from build123d import *

# Parameters (mm, degrees)
SKETCH1_R           = 38
BOSS_EXTRUDE1_DEPTH = 10
SKETCH2_R           = 2.5
CUT_EXTRUDE1_DEPTH  = 10
CIRPATTERN1_COUNT   = 8


with BuildPart() as part:
    # Sketch1 → Boss-Extrude1 (new body)
    with BuildSketch(Plane.XY):
        Circle(SKETCH1_R)
    extrude(amount=BOSS_EXTRUDE1_DEPTH)

    # Sketch2 → Cut-Extrude1 (cut)
    with BuildSketch(Plane(origin=(0, 38, 0), x_dir=(1, 0, 0), z_dir=(0, 1, 0))):
        with Locations((0, -5)):
            Circle(SKETCH2_R)
    cut_extrude1 = extrude(amount=-CUT_EXTRUDE1_DEPTH, mode=Mode.SUBTRACT)

    # CirPattern1: Cut-Extrude1 ×8 about axis
    cirpattern1_axis = Axis((0, 0, 0), (0, 0, 1))
    for i in range(1, CIRPATTERN1_COUNT):
        add(cut_extrude1.rotate(cirpattern1_axis, i * 360 / CIRPATTERN1_COUNT), mode=Mode.SUBTRACT)


solid = part.part
Verification items for the finished model (mm, model axes). A direction names the side the tool comes from. Give positions to 0.01 mm unless a question says otherwise; leave off trailing zeros. Order: outer loops, then holes, each group sorted by start corner. A loop starts at its lowest first (then second) coordinate and runs counter-clockwise, first axis right, second up. Notation, with made-up numbers: M 1,9.5 L 22,9.5 A17 ccw 22,35.5 Z; hole C 44,53 d8. An arc over 180 degrees is marked long. Answer as a JSON object with one key per item and string values. Group by question number.
1) Cross-section at A-A (y = 0). Enter the section's corners in (x, z), then the cut area to 3 significant figures.
2) Depth check by flat-ended pin: pin 1 Ø1.5 at (y, z) = (1, 4) entering from -X; pin 2 Ø2.5 at (x, z) = (0.5, 4.5) entering from +Y; pin 3 Ø5 at (x, z) = (15, 5.5) entering from -Y. Enter the tip coordinate at first touch or a pass-through.
3) Scan lines: line 1 along Z through (x, y) = (-31, 0); line 2 along X through (y, z) = (-33.5, 7.25); line 3 along Y through (x, z) = (-30.5, 2.75). Record each from-to range of solid material in increasing order. Write a range as [from, to].
4) Mould release check, pull along X, two halves, no side actions. Record for faces 1 (the face through (35.102, -14.554, 4.93)), 2 (the face through (-24.33, -22.43, 2.89)), 3 (the face through (-28, 0, 5)): released by +X, released by -X, zero draft, split by the parting line, or undercut.
5) Access from +Z, -Z, +X, -X, +Y, -Y to the whole of each face (thin tool, end or side, straight path). Record for faces 4 (the face through (-0.33, 33.07, 2.52)), 5 (the face through (0.33, -33.07, 2.52)), 6 (the face through (-19.8, 19.8, 5)), 7 (the face through (-33.07, -0.33, 2.52)), 8 (the face through (28, 0, 5)).
6) Cross-section at D-D (x = -30). Enter the section's corners in (y, z).
Result sheet:
{
 "1": {"outline": "M -38,0 L 38,0 L 38,2.5 L 28,2.5 L 28,7.5 L 38,7.5 L 38,10 L -38,10 L -38,7.5 L -28,7.5 L -28,2.5 L -38,2.5 Z", "area": "660 mm2"},
 "2": {"pin 1": "stops at x = -28", "pin 2": "stops at y = 28", "pin 3": "stops at y = -35.89"},
 "3": {"line 1": "z = [0, 2.5], [7.5, 10]", "line 2": "x = [-17.94, -1.09], [1.09, 17.94]", "line 3": "y = [-22.67, -1.09], [1.09, 22.67]"},
 "4": {"face 1": "split by the parting line", "face 2": "undercut", "face 3": "released by -X"},
 "5": {"face 4": "+Y", "face 5": "-Y", "face 6": "none", "face 7": "-X", "face 8": "+X"},
 "6": {"outline": "M -23.32,0 L 23.32,0 L 23.32,10 L -23.32,10 Z; hole C 0,5 d5"}
}
